Model file for the job. Use its own axes, mm. Round coordinates to 2 decimals unless told otherwise and drop trailing zeros. Loops run counter-clockwise (first coordinate to the right, second up) from the corner with the lowest first, then second, coordinate; pieces in that order, holes last. Notation, with made-up numbers: (53.5, 28) - (73.5, 28) arc R16 cw to (73.5, 59) - close; hole circle Ø5 at (78.25, -37.5). An arc over 180 degrees is marked (long way). Use one line per item in the form item = value.
from build123d import *

# Parameters (mm, degrees)
SKETCH1_R                                    = 40
SKETCH1_R_2                                  = 22
BOSS_EXTRUDE1_DEPTH                          = 6
CSK_FOR_M5_COUNTERSUNK_FLAT_HEAD_SCR_2_COUNT = 2
CSK_FOR_M5_COUNTERSUNK_FLAT_HEAD_SCR_2_PITCH = 45.961940777
CSK_FOR_M5_COUNTERSUNK_FLAT_HEAD_SCR_3_COUNT = 2
CSK_FOR_M5_COUNTERSUNK_FLAT_HEAD_SCR_3_PITCH = 65
CSK_FOR_M5_COUNTERSUNK_FLAT_HEAD_SCR_4_COUNT = 2
CSK_FOR_M5_COUNTERSUNK_FLAT_HEAD_SCR_4_PITCH = 45.961940777


with BuildPart() as part:
    # Sketch1 → Boss-Extrude1 (new body)
    with BuildSketch(Plane.XY):
        Circle(SKETCH1_R)
        Circle(SKETCH1_R_2, mode=Mode.SUBTRACT)
    extrude(amount=BOSS_EXTRUDE1_DEPTH)

    # Sketch6 → CSK for M5 Countersunk Flat Head Screw1 (revolve, cut)
    with BuildSketch(Plane(origin=(0, 32.5, 6), x_dir=(0, -1, 0), z_dir=(1, 0, 0))):
        Polygon((0, 0), (0, 6), (3.3, 6), (3.3, 3.42), (6.72, 0), align=None)
    csk_for_m5_countersunk_flat_head_screw1 = revolve(axis=Axis((0, 32.5, 12.35), (0, 0, -1)), mode=Mode.SUBTRACT)

    # CSK for M5 Countersunk Flat Head Scr 2: CSK for M5 Countersunk Flat Head Screw1 ×2
    with Locations(*[Vector(-0.7071067811865476, -0.7071067811865476, 0) * (i * CSK_FOR_M5_COUNTERSUNK_FLAT_HEAD_SCR_2_PITCH) for i in range(1, CSK_FOR_M5_COUNTERSUNK_FLAT_HEAD_SCR_2_COUNT)]):
        add(csk_for_m5_countersunk_flat_head_screw1, mode=Mode.SUBTRACT)

    # CSK for M5 Countersunk Flat Head Scr 3: CSK for M5 Countersunk Flat Head Screw1 ×2
    with Locations(*[(0, -i * CSK_FOR_M5_COUNTERSUNK_FLAT_HEAD_SCR_3_PITCH, 0) for i in range(1, CSK_FOR_M5_COUNTERSUNK_FLAT_HEAD_SCR_3_COUNT)]):
        add(csk_for_m5_countersunk_flat_head_screw1, mode=Mode.SUBTRACT)

    # CSK for M5 Countersunk Flat Head Scr 4: CSK for M5 Countersunk Flat Head Screw1 ×2
    with Locations(*[Vector(0.7071067811865476, -0.7071067811865476, 0) * (i * CSK_FOR_M5_COUNTERSUNK_FLAT_HEAD_SCR_4_PITCH) for i in range(1, CSK_FOR_M5_COUNTERSUNK_FLAT_HEAD_SCR_4_COUNT)]):
        add(csk_for_m5_countersunk_flat_head_screw1, mode=Mode.SUBTRACT)


solid = part.part
1. Flat gauge pins, fed straight in: pin 1 (7.5 mm diameter, centred on x = 32.5, y = 0, fed in from +Z); pin 2 (8.5 mm diameter, centred on x = -32.5, y = 0, fed in from +Z); pin 3 (1.5 mm diameter, centred on x = 17.5, z = 1.5, fed in from -Y). Where does each tip first touch, or does it go through?
Geometry check:
pin_1 = 3.03
pin_2 = 3.53
pin_3 = -36.32
2. Cut at D-D, the plane z = 5. Give the cut face in (x, y), plus the area to 3 significant figures.
Geometry check:
outline = circle Ø80 at (0, 0); hole circle Ø11.44 at (-32.5, 0); hole circle Ø44 at (0, 0); hole circle Ø11.44 at (0, -32.5); hole circle Ø11.44 at (0, 32.5); hole circle Ø11.44 at (32.5, 0)
area = 3,090 mm^2
3. Wall check: probe 1 along Y at (x, z) = (0, 1.7); probe 2 along X at (y, z) = (-1.5, 1.9); probe 3 along X at (y, z) = (-1, 3.4). Give the ranges that are in metal, low to high.
Geometry check:
probe_1 = -40 to -35.8, -29.2 to -22, 22 to 29.2, 35.8 to 40
probe_2 = -39.97 to -35.44, -29.56 to -21.95, 21.95 to 29.56, 35.44 to 39.97
probe_3 = -39.99 to -36.5, -28.5 to -21.98, 21.98 to 28.5, 36.5 to 39.99
4. Pull direction X, two halves, no side cores. Call faces 1 (the cylindrical face through (-35.77, 0.43, 1.31)), 2 (the flat face through (17, -17, 6)), 3 (the cylindrical face through (-8.67, -39.05, 2.96)): +X half, -X half, draft (parallel to the pull), parting line (faces both ways), or undercut.
Geometry check:
face_1 = undercut
face_2 = draft
face_3 = parting line
5. Cut at A-A, the plane y = 0. Give the cut face in (x, z), plus the area to 3 significant figures.
Geometry check:
outline = (-40, 0) - (-35.8, 0) - (-35.8, 2.58) - (-39.22, 6) - (-40, 6) - close; (-29.2, 0) - (-22, 0) - (-22, 6) - (-25.78, 6) - (-29.2, 2.58) - close; (22, 0) - (29.2, 0) - (29.2, 2.58) - (25.78, 6) - (22, 6) - close; (35.8, 0) - (40, 0) - (40, 6) - (39.22, 6) - (35.8, 2.58) - close
area = 113 mm^2
6. Cut at C-C, the plane y = -11. Give the cut face in (x, z).
Geometry check:
outline = (-38.46, 0) - (-19.05, 0) - (-19.05, 6) - (-38.46, 6) - close; (19.05, 0) - (38.46, 0) - (38.46, 6) - (19.05, 6) - close
